Part model, mm, in its own coordinate system. A direction names the side the tool comes from. Round coordinates to 2 decimals unless told otherwise and drop trailing zeros. Loops run counter-clockwise (first coordinate to the right, second up) from the corner with the lowest first, then second, coordinate; pieces in that order, holes last. Notation, with made-up numbers: M 23,-23 L 70,-23 A17 ccw 70,-12 Z; hole C -8.5,-34 d1. An arc over 180 degrees is marked long. Put each result on its own line as item: value. Start each with the question number.
1) Slice it at A-A on y = 23. Give the cut face in (x, z) (3 decimals).
2) Which spindle directions (+Z, -Z, +X, -X, +Y, -Y) get a long thin tool onto all of the face, cutting with end or side? Do faces 1 (the flat face through (-28.575, 6, 0)), 2 (the flat face through (0, 0, 0)). Say none if no direction does.
3) Slice it at D-D on z = 9.5. Give the cut face in (x, y) (3 decimals), then the cut area to 3 significant figures.
4) Drop a flat-ended pin along its axis: pin 1 Ø12 at (x, z) = (-9, -8.5) entering from +Y. Give the stop position or say it passes through.
5) Slice it at B-B on z = 0. State how many separate pieces and enclosed holes the cut face has, then the cut area to 3 significant figures.
6) Pull direction Z, two halves, no side cores. Call faces 3 (the cylindrical face through (-25.44, 8.05, -1.03)), 4 (the flat face through (0, -1, 12.7)), 5 (the flat face through (-25, 25.4, 0)), 6 (the flat face through (0, -1, -12.7)): +Z half, -Z half, draft (parallel to the pull), parting line (faces both ways), or undercut.
7) Slice it at C-C on y = 12.7. Give the cut face in (x, z) (1 decimal), then the cut area to 3 significant figures.
8) Probe line 1 along X through (y, z) = (9, -8.75) (3 decimals); line 2 along Y through (x, z) = (-25.75, 0); line 3 along Z through (x, y) = (25, 12.7). List the from-to ranges inside material, lowest first.
Autodesk Inventor part; units mm, degrees
ref_plane "XZ Plane" through (0, 0, 0) normal (0, 1, 0) x (-1, 0, 0)
sketch "Sketch1" plane through (0, 0, 0) normal (0, 1, 0) x (-1, 0, 0)
  line L0 (28.575, 12.7) -> (-28.575, 12.7)
  line L1 (-28.575, 12.7) -> (-28.575, -12.7)
  line L2 (-28.575, -12.7) -> (28.575, -12.7)
  line L3 (28.575, -12.7) -> (28.575, 12.7)
  line L4 (28.575, 12.7) -> (-28.575, -12.7) construction
  line L5 (-28.575, 12.7) -> (28.575, -12.7) construction
  point P0 (0, 0)
  dimension "d0" = 57.15
  dimension "d1" = 25.4
extrude "Extrusion1" add sketch "Sketch1" against normal blind 6.35
sketch "Sketch2" plane through (0, 0, 0) normal (0, 1, 0) x (1, 0, 0)
  line L0 (-28.575, -12.7) -> (-28.575, 12.7)
  line L1 (-28.575, -12.7) -> (-22.225, -12.7)
  line L2 (-22.225, -12.7) -> (-22.225, 12.7)
  line L3 (-22.225, 12.7) -> (-28.575, 12.7)
  line L4 (-28.575, 12.7) -> (-28.575, -12.7)
  point P0 (0, 0)
  dimension "d4" = 6.35
extrude "Extrusion2" add sketch "Sketch2" along normal blind 25.4
sketch "Sketch3" plane through (-28.575, -6.35, -12.7) normal (-1, 0, 0) x (0, 0, 1)
  circle A0 centre (12.7, 19.05) radius 4.7625
  line L0 (0, 31.75) -> (25.4, 31.75)
  circle A1 centre (12.7, -19.05) radius 4.0284
  point P0 (12.7, 6.35)
  dimension "d7" = 9.525
  dimension "d8" = 12.7
  dimension "d11" = 50.8
extrude "Extrusion3" cut sketch "Sketch3" against normal through all contours A0
mirror "Mirror1" about plane through (0, 0, 0) normal (1, 0, 0) of "Extrusion2", "Extrusion3"
properties part number "camPostHolderV02"
Recorded:
1. outline: M -28.575,-12.7 L -22.225,-12.7 L -22.225,12.7 L -28.575,12.7 Z; M 22.225,-12.7 L 28.575,-12.7 L 28.575,12.7 L 22.225,12.7 Z
2. face 1: +Z, -Z, -X, +Y, -Y
2. face 2: +Z, -Z, +Y
3. outline: M -28.575,-6.35 L 28.575,-6.35 L 28.575,25.4 L 22.225,25.4 L 22.225,0 L -22.225,0 L -22.225,25.4 L -28.575,25.4 Z
3. area: 685 mm2
4. pin 1: stops at y = 0
5. separate pieces: 3
5. enclosed holes: 0
5. area: 565 mm2
6. face 3: undercut
6. face 4: +Z half
6. face 5: draft
6. face 6: -Z half
7. outline: M -28.6,-12.7 L -22.2,-12.7 L -22.2,-4.8 L -28.6,-4.8 Z; M -28.6,4.8 L -22.2,4.8 L -22.2,12.7 L -28.6,12.7 Z; M 22.2,-12.7 L 28.6,-12.7 L 28.6,-4.8 L 22.2,-4.8 Z; M 22.2,4.8 L 28.6,4.8 L 28.6,12.7 L 22.2,12.7 Z
7. area: 202 mm2
8. line 1: x = -28.575 to -22.225, 22.225 to 28.575
8. line 2: y = -6.35 to 7.94, 17.46 to 25.4
8. line 3: z = -12.7 to -4.76, 4.76 to 12.7
